from build123d import *

# Parameters (mm, degrees)
SKETCH1_R           = 5.5
BOSS_EXTRUDE1_DEPTH = 20
SKETCH2_R           = 7
BOSS_EXTRUDE2_DEPTH = 5
CHAMFER2_SIZE       = 2
SKETCH3_R           = 2
CUT_EXTRUDE1_DEPTH  = 10
SKETCH6_W           = 14.643635598
SKETCH6_H           = 6.4
CUT_EXTRUDE2_DEPTH  = 3
CHAMFER4_SIZE       = 1
MIRROR4_START       = -20
MIRROR4_2_DEPTH     = 3
MIRROR4_START_2     = -17
MIRROR4_3_OUTLINE_R = 2
MIRROR4_3_DEPTH     = 2


# Read off the part's stored shape, not the designer's step: Mirror4
with BuildPart() as part:
    # Sketch1 → Boss-Extrude1 (new, symmetric)
    with BuildSketch(Plane(origin=(0, 0, 0), x_dir=(1, 0, 0), z_dir=(0, 1, 0))):
        with Locations(Location((0, 0, 0), (0, 0, 270))):
            Circle(SKETCH1_R)
    extrude(amount=BOSS_EXTRUDE1_DEPTH, both=True)

    # Sketch2 → Boss-Extrude2 (add)
    with BuildSketch(Plane(origin=(0, 20, 0), x_dir=(1, 0, 0), z_dir=(0, 1, 0))):
        with Locations(Location((0, 0, 0), (0, 0, 270))):
            Circle(SKETCH2_R)
    extrude(amount=BOSS_EXTRUDE2_DEPTH)

    # Chamfer2
    # the kernel refuses this chamfer: 2 mm, written as the material it takes off along each edge
    with BuildSketch(Plane(origin=(0, 20, 0), x_dir=(0, 0, 1), z_dir=(-1, 0, 0))) as chamfer2_piece_1_section:
        Polygon((7, CHAMFER2_SIZE), (7 - CHAMFER2_SIZE, 0), (7, 0), align=None)
    chamfer2_piece_1 = revolve(axis=Axis((0, 20, 0), (0, 1, 0)), mode=Mode.PRIVATE)
    chamfer2_piece_1 = chamfer2_piece_1 - Plane(origin=(0, 21.24754516, 0), x_dir=(0, 0, 1), z_dir=(0, 1, 0)) * Cylinder(5.5, 28, mode=Mode.PRIVATE)
    add(chamfer2_piece_1, mode=Mode.SUBTRACT)

    # Sketch3 → Cut-Extrude1 (cut)
    with BuildSketch(Plane(origin=(0, 25, 0), x_dir=(1, 0, 0), z_dir=(0, 1, 0))):
        with Locations(Location((0, 0, 0), (0, 0, 270))):
            Circle(SKETCH3_R)
    extrude(amount=-CUT_EXTRUDE1_DEPTH, mode=Mode.SUBTRACT)

    # Sketch6 → Cut-Extrude2 (cut)
    with BuildSketch(Plane(origin=(0, 20, 0), x_dir=(-1, 0, 0), z_dir=(0, -1, 0))):
        with Locations((-3.821817799, 0)):
            Rectangle(SKETCH6_W, SKETCH6_H)
    extrude(amount=CUT_EXTRUDE2_DEPTH, mode=Mode.SUBTRACT)

    # Chamfer4
    chamfer4_edges = [part.edges().sort_by_distance(p)[0] for p in [
        (-3.5, 18.5, -3.2),
        (-3.5, 18.5, 3.2),
    ]]
    chamfer(chamfer4_edges, length=CHAMFER4_SIZE)

    # Mirror4 outline → Mirror4 (revolve)
    with BuildSketch(Plane.XY):
        Polygon((7, -25), (7, -22), (5.5, -20.5), (5.5, -20), (2, -20), (2, -25), align=None)
    revolve(axis=Axis((0, 0, 0), (0, 1, 0)))

    # Mirror4 2 outline → Mirror4 2 (cut)
    with BuildSketch(Plane(origin=(0, 0, 0), x_dir=(1, 0, 0), z_dir=(0, 1, 0)).offset(MIRROR4_START)):
        with BuildLine():
            Line((4.473253849, 3.2), (-2.5, 3.2))
            Line((-2.5, 3.2), (-3.5, 2.2))
            Line((-3.5, 2.2), (-3.5, -2.2))
            Line((-3.5, -2.2), (-2.5, -3.2))
            Line((-2.5, -3.2), (4.473253849, -3.2))
            ThreePointArc((4.473253849, -3.2), (5.5, 0), (4.473253849, 3.2))
        make_face()
    extrude(amount=MIRROR4_2_DEPTH, mode=Mode.SUBTRACT)

    # Mirror4 3 outline → Mirror4 3 (cut)
    with BuildSketch(Plane(origin=(0, 0, 0), x_dir=(1, 0, 0), z_dir=(0, 1, 0)).offset(MIRROR4_START_2)):
        Circle(MIRROR4_3_OUTLINE_R)
    extrude(amount=MIRROR4_3_DEPTH, mode=Mode.SUBTRACT)


solid = part.part
Input: part model. Units: mm. Frame: model coordinates. A direction names the side the tool comes from. Coordinates: 2 decimals unless noted, no trailing zeros. Order: outer loops, then holes, each group sorted by start corner. A loop starts at its lowest first (then second) coordinate and runs counter-clockwise, first axis right, second up.
1. Cut plane D-D, the plane y = 10. Return loops of the section in (x, z), plus the area to 3 significant figures.
Checked values:
outline: circle Ø11 at (0, 0)
area: 95.0 mm2
2. Cut plane B-B, the plane z = -1.5. Count the separate pieces of the cut face and the enclosed holes in it, plus the area to 3 significant figures.
Checked values:
separate pieces: 3
enclosed holes: 0
area: 463 mm2
3. Contact query for flat-ended pins moving along their axis: P1, Ø1.2, axis at x = 0.5, z = 0, coming from the +Y side; P2, Ø3.5, axis at x = 1, y = 19, coming from the -Z side; P3, Ø8, axis at x = 0, y = 0, coming from the +Z side. Output: stop coordinate, or through.
Checked values:
P1: stops at y = 15
P2: stops at z = -5.68
P3: stops at z = 5.5
4. Cut plane C-C, the plane y = -18.5. Return loops of the section in (x, z).
Checked values:
outline: (-3.5, -2.2) - (-3.5, 2.2) - (-2.5, 3.2) - (4.47, 3.2) arc R5.5 ccw (long way) to (4.47, -3.2) - (-2.5, -3.2) - close
5. Draft query along Z for faces 1 (the flat face through (2, 25, 1)), 2 (the conical face through (-6, -21, 0)), 3 (the flat face through (1, -19, 3.2)). Return one class per face: +Z half, -Z half, draft (parallel to the pull), parting line (faces both ways), or undercut.
Checked values:
face 1: draft
face 2: parting line
face 3: undercut
6. Access query for faces 4 (the cylindrical face through (-2, 23, 0)), 5 (the cylindrical face through (0, -23, 2)), 6 (the flat face through (2, -20, 1)), 7 (the flat face through (-1, -25, -2)). Directions: +Z, -Z, +X, -X, +Y, -Y. A direction counts if a zero-diameter tool reaches every point of the face in a straight line with its end or side. Return the directions, or none.
Checked values:
face 4: +Y
face 5: -Y
face 6: +X
face 7: +Z, -Z, +X, -X, -Y
7. Cut plane A-A, the plane y = 16. Return loops of the section in (x, z), plus the area to 3 significant figures.
Checked values:
outline: circle Ø11 at (0, 0); hole circle Ø4 at (0, 0)
area: 82.5 mm2
8. Ray query, line 1 along Y through (x, z) = (4.75, 2.5); line 2 along Z through (x, y) = (0, -22.1); line 3 along Y through (x, z) = (5.25, -2.5). Return the intervals inside material, ascending.
Checked values:
line 1: y = -25 to -20, -17 to 17, 20 to 25
line 2: z = -7 to -2, 2 to 7
line 3: y = -25 to -20.81, 20.81 to 25
